Read the model definition and answer for the solid it produces. Units are mm, in the model's axes. Face numbers are marked on the shaded views. A direction names the side the tool comes from. Round coordinates to 2 decimals unless told otherwise and drop trailing zeros. Write each loop counter-clockwise with the first axis right and the second up, starting at its lowest first coordinate (ties: lowest second). Pieces come first, ordered by that corner, then holes. Notation, with made-up numbers: (-14.75, -33.5) - (0.25, -33.5) arc R16 cw to (0.25, -29.5) - close; hole circle Ø2 at (39.25, -9.75). An arc over 180 degrees is marked (long way). Use one line per item in the form item = value. Start each with the question number.
1) The part is cut by section C-C, the plane x = 9. Give the vertices of the cut face in (y, z) (3 decimals), plus the area to 3 significant figures.
2) The part is cut by section B-B, the plane z = 3.5. Give the vertices of the cut face in (x, y), plus the area to 3 significant figures.
3) The part is cut by section A-A, the plane y = -7.5. Give the vertices of the cut face in (x, z) (3 decimals).
4) For a pull along Y with two mould halves and no side action, classify the marked faces 1, 2 and 3 as released by +Y, released by -Y, zero draft, split by the parting line, or undercut.
5) Each of these flat-tipped pins is pushed along its axis until it touches: pin 1 (1 mm diameter, centred on y = -7.5, z = 10, fed in from +X); pin 2 (5 mm diameter, centred on x = 9, y = -7.5, fed in from -Z); pin 3 (2 mm diameter, centred on y = -6, z = 14.5, fed in from +X); pin 4 (4 mm diameter, centred on x = 9, y = -7.5, fed in from +Z) (3 decimals). Where does it stop, or does it pass through?
6) The part is cut by section D-D, the plane x = 12.5. Give the vertices of the cut face in (y, z) (3 decimals), plus the area to 3 significant figures.
7) For the marked faces 4, 5 and 6, determine the directions among +Z, -Z, +X, -X, +Y, -Y from which every point of the face is accessible in a straight line to the end or side of a thin tool.
8) Consider line 1 along Y through (x, z) = (9, 4.5); line 2 along Z through (x, y) = (6.25, -10.5) (3 decimals); line 3 along X through (y, z) = (-5.75, 10.75). Determine where each line is inside the solid, lowest interval first. Write a range as from..to.
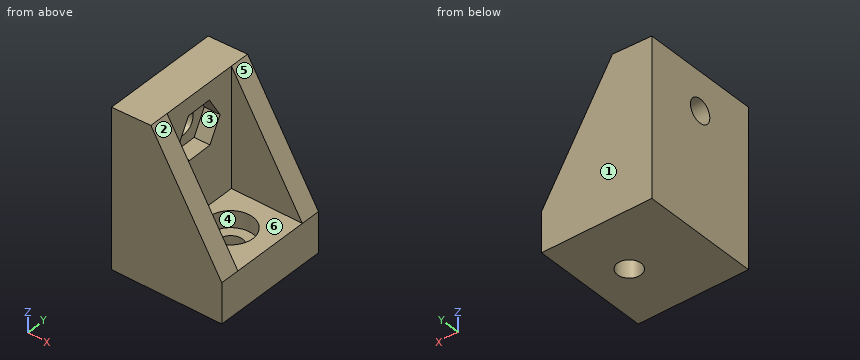
from build123d import *

# Parameters (mm, degrees)
F1_DEPTH       = 15
F2_DEPTH       = 2.5
F5_DEPTH       = 2.5
F7_D           = 3
F7_CBORE_D     = 5.6
F7_CBORE_DEPTH = 2.1
F9_D           = 3
F10_DEPTH      = 2


with BuildPart() as f1:
    # F0 (on Front) → F1 (new body)
    with BuildSketch(Plane.XZ):
        Polygon((4.9977494935, 20.15), (0, 20), (0, 0), (14, 0), (14, 5.075), (4.9977494935, 5.075), align=None)
    extrude(amount=F1_DEPTH)

    # F0 (on Front) → F2 (join)
    with BuildSketch(Plane.XZ):
        Polygon((4.9977494935, 20.15), (0, 20), (0, 0), (14, 0), (14, 5.075), (4.9977494935, 5.075), align=None)
        Polygon((14, 5.075), (4.9977494935, 20.15), (4.9977494935, 5.075), align=None)
    extrude(amount=F2_DEPTH)

    # F4 (on offset) → F5 (join)
    with BuildSketch(Plane.XZ.offset(15)):
        Polygon((14, 5.075), (4.9977494935, 20.15), (4.9977494935, 5.075), align=None)
    extrude(amount=-F5_DEPTH)

    # F7 (through all)
    with Locations(Plane.XY.offset(5.075)):
        with Locations((9, -7.5)):
            CounterBoreHole(F7_D / 2, F7_CBORE_D / 2, F7_CBORE_DEPTH)

    # F9 (through all)
    with Locations(Plane.YZ.offset(4.9977494935)):
        with Locations((-7.5, 15.15)):
            Hole(F9_D / 2)

    # F8 (on face) → F10 (cut)
    with BuildSketch(Plane.YZ.offset(4.9977494935)):
        Polygon((-9.1603395536, 17.9242757433), (-10.7327630476, 15.0992416393), (-9.072423494, 12.324965896), (-5.8396604464, 12.3757242567), (-4.2672369524, 15.2007583607), (-5.927576506, 17.975034104), align=None)
    extrude(amount=-F10_DEPTH, mode=Mode.SUBTRACT)


solid = f1.part
Geometry results:
q1.outline = (-15, 0) - (-9, 0) - (-9, 2.975) - (-10.3, 2.975) - (-10.3, 5.075) - (-12.5, 5.075) - (-12.5, 13.448) - (-15, 13.448) - close; (-6, 0) - (0, 0) - (0, 13.448) - (-2.5, 13.448) - (-2.5, 5.075) - (-4.7, 5.075) - (-4.7, 2.975) - (-6, 2.975) - close
q1.area = 97.3 mm2
q2.outline = (0, -15) - (14, -15) - (14, 0) - (0, 0) - close; hole circle Ø5.6 at (9, -7.5)
q2.area = 185 mm2
q3.outline = (0, 0) - (7.5, 0) - (7.5, 2.975) - (6.2, 2.975) - (6.2, 5.075) - (4.998, 5.075) - (4.998, 12.35) - (2.998, 12.35) - (2.998, 13.65) - (0, 13.65) - close; (0, 16.65) - (2.998, 16.65) - (2.998, 17.95) - (4.998, 17.95) - (4.998, 20.15) - (0, 20) - close; (10.5, 0) - (14, 0) - (14, 5.075) - (11.8, 5.075) - (11.8, 2.975) - (10.5, 2.975) - close
q4.face_1 = released by +Y
q4.face_2 = zero draft
q4.face_3 = undercut
q5.pin_1 = 5
q5.pin_2 = 0
q5.pin_3 = 3
q5.pin_4 = 2.975
q6.outline = (-15, 0) - (0, 0) - (0, 7.587) - (-2.5, 7.587) - (-2.5, 5.075) - (-12.5, 5.075) - (-12.5, 7.587) - (-15, 7.587) - close
q6.area = 88.7 mm2
q7.face_4 = +Z
q7.face_5 = +Z, +X, +Y, -Y
q7.face_6 = +Z, +X
q8.line_1 = -15..-10.3, -4.7..0
q8.line_2 = 0..5.075
q8.line_3 = 0..5
